Design review of the part built by this model. Coordinates are the model's own, in mm. Face numbers are marked on the shaded views. A direction names the side the tool comes from. Coordinates: 2 decimals unless noted, no trailing zeros. Write each loop counter-clockwise with the first axis right and the second up, starting at its lowest first coordinate (ties: lowest second). Pieces come first, ordered by that corner, then holes. Notation, with made-up numbers: (24.5, 7.5) -> (32.5, 7.5) arc R4 cw to (32.5, 14.5) -> close; hole circle Ø8 at (44.5, 51). An arc over 180 degrees is marked (long way). One line per question, with ' | ' between items. Start each with the question number.
Q1. Add section B-B on y = 2.5. State the section outline as (x, z) points.
Q2. For P1, Ø0.6, axis at x = 12, z = 3, coming from the -Y side (3 decimals); P2, Ø1.6, axis at y = 5, z = 1.5, coming from the +X side; P3, Ø1, axis at x = 2.85, y = 2, coming from the -Z side; P4, Ø2, axis at x = 13.35, y = 2, coming from the +Z side, all flat-tipped, find the tip position at first contact; note any pin that passes through.
Q3. Add section D-D on x = 1.75. State the section outline as (y, z) points (3 decimals).
Q4. Draft analysis for pull direction Y (two halves, no side actions). For the marked faces 5, 6, 7 and 8, state which applies: pulls with the +Y half, pulls with the -Y half, needs draft (parallel to the pull), parting line crosses it, or undercut.
Q5. Wall thickness on probe 1 along X at (y, z) = (8, 0.75); probe 2 along X at (y, z) = (11.75, 1.7); probe 3 along Y at (x, z) = (13.35, 0.75): over which ranges is each line inside the solid? List them lowest first.
Q6. For the marked faces 1, 2, 3 and 4, list the 3-axis set-ups (+Z, -Z, +X, -X, +Y, -Y) from which the entire face can be reached by the end or side of a thin tool; tool diameter is ignored.
Q7. Add section C-C on z = 1.4. State the section outline as (x, y) points (3 decimals).
Q8. Add section A-A on x = 13.35. State the section outline as (y, z) points (3 decimals).
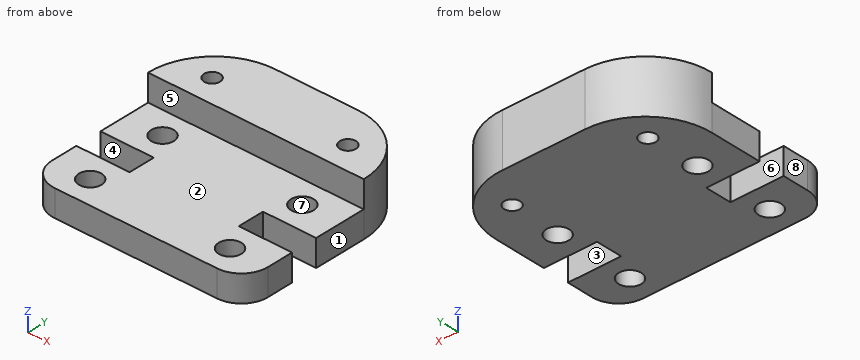
from build123d import *

# Parameters (mm, degrees)
SKETCH2_R           = 0.85
SKETCH2_R_2         = 0.6
BOSS_EXTRUDE1_DEPTH = 4
SKETCH3_W           = 16.2
SKETCH3_H           = 9.945
CUT_EXTRUDE2_DEPTH  = 2


with BuildPart() as part:
    # Sketch2 → Boss-Extrude1 (new body)
    with BuildSketch(Plane.XY):
        with BuildLine():
            Line((0, 9.945), (0, 6))
            Line((0, 6), (4, 6))
            Line((4, 6), (4, 4))
            Line((4, 4), (0, 4))
            Line((0, 4), (0, 2))
            ThreePointArc((0, 2), (0.585786438, 0.585786438), (2, 0))
            Line((2, 0), (14.2, 0))
            ThreePointArc((14.2, 0), (15.614213562, 0.585786438), (16.2, 2))
            Line((16.2, 2), (16.2, 4))
            Line((16.2, 4), (12.2, 4))
            Line((12.2, 4), (12.2, 6))
            Line((12.2, 6), (16.2, 6))
            Line((16.2, 6), (16.2, 9.945))
            ThreePointArc((16.2, 9.945), (14.735533906, 13.480533906), (11.2, 14.945))
            Line((11.2, 14.945), (5, 14.945))
            ThreePointArc((5, 14.945), (1.464466094, 13.480533906), (0, 9.945))
        make_face()
        with Locations((13.35, 8)):
            Circle(SKETCH2_R, mode=Mode.SUBTRACT)
        with Locations((13.35, 2)):
            Circle(SKETCH2_R, mode=Mode.SUBTRACT)
        with Locations((13.2, 11.942)):
            Circle(SKETCH2_R_2, mode=Mode.SUBTRACT)
        with Locations((3, 11.942)):
            Circle(SKETCH2_R_2, mode=Mode.SUBTRACT)
        with Locations((2.85, 2)):
            Circle(SKETCH2_R, mode=Mode.SUBTRACT)
        with Locations((2.85, 8)):
            Circle(SKETCH2_R, mode=Mode.SUBTRACT)
    extrude(amount=BOSS_EXTRUDE1_DEPTH)

    # Sketch3 → Cut-Extrude2 (cut)
    with BuildSketch(Plane(origin=(0, 0, 4), x_dir=(-1, 0, 0), z_dir=(0, 0, -1))):
        with Locations((-8.1, 4.9725)):
            Rectangle(SKETCH3_W, SKETCH3_H)
    extrude(amount=CUT_EXTRUDE2_DEPTH, mode=Mode.SUBTRACT)


solid = part.part
Output values:
1) outline: (0, 0) -> (2.16, 0) -> (2.16, 2) -> (0, 2) -> close; (3.54, 0) -> (12.66, 0) -> (12.66, 2) -> (3.54, 2) -> close; (14.04, 0) -> (16.2, 0) -> (16.2, 2) -> (14.04, 2) -> close
2) P1: stops at y = 9.945 | P2: stops at x = 12.2 | P3: passes through | P4: stops at z = 2
3) outline: (0.016, 0) -> (4, 0) -> (4, 2) -> (0.016, 2) -> close; (6, 0) -> (13.745, 0) -> (13.745, 4) -> (9.945, 4) -> (9.945, 2) -> (6, 2) -> close
4) face 5: pulls with the -Y half | face 6: undercut | face 7: undercut | face 8: needs draft
5) probe 1: x = 0 to 2, 3.7 to 12.5, 14.2 to 16.2 | probe 2: x = 0.34 to 2.43, 3.57 to 12.63, 13.77 to 15.86 | probe 3: y = 0 to 1.15, 2.85 to 4, 6 to 7.15, 8.85 to 11.36, 12.52 to 14.46
6) face 1: +Z, -Z, +X, +Y, -Y | face 2: +Z, +X, -X, -Y | face 3: +Z, -Z, +X | face 4: +Z, -Z, -X
7) outline: (0, 2) arc R2 ccw to (2, 0) -> (14.2, 0) arc R2 ccw to (16.2, 2) -> (16.2, 4) -> (12.2, 4) -> (12.2, 6) -> (16.2, 6) -> (16.2, 9.945) arc R5 ccw to (11.2, 14.945) -> (5, 14.945) arc R5 ccw to (0, 9.945) -> (0, 6) -> (4, 6) -> (4, 4) -> (0, 4) -> close; hole circle Ø1.7 at (2.85, 2); hole circle Ø1.7 at (2.85, 8); hole circle Ø1.2 at (3, 11.942); hole circle Ø1.7 at (13.35, 2); hole circle Ø1.7 at (13.35, 8); hole circle Ø1.2 at (13.2, 11.942)
8) outline: (0, 0) -> (1.15, 0) -> (1.15, 2) -> (0, 2) -> close; (2.85, 0) -> (4, 0) -> (4, 2) -> (2.85, 2) -> close; (6, 0) -> (7.15, 0) -> (7.15, 2) -> (6, 2) -> close; (8.85, 0) -> (11.361, 0) -> (11.361, 4) -> (9.945, 4) -> (9.945, 2) -> (8.85, 2) -> close; (12.523, 0) -> (14.459, 0) -> (14.459, 4) -> (12.523, 4) -> close
